from build123d import *

# Parameters (mm, degrees)
BOSS_EXTRUDE1_DEPTH = 50
BOSS_EXTRUDE2_DEPTH = 1.52
CUT_EXTRUDE2_DEPTH  = 1.52
CUT_EXTRUDE3_DEPTH  = 29
BOSS_EXTRUDE3_DEPTH = 1.55
SKETCH6_R           = 1
CUT_EXTRUDE4_DEPTH  = 77.55
CUT_EXTRUDE5_DEPTH  = 77.55
SKETCH8_R           = 1
CUT_EXTRUDE6_DEPTH  = 70
BOSS_EXTRUDE4_DEPTH = 1.5
BOSS_EXTRUDE5_DEPTH = 1.5
SKETCH12_R          = 10
CUT_EXTRUDE7_DEPTH  = 70


with BuildPart() as part:
    # Sketch1 → Boss-Extrude1 (new body)
    with BuildSketch(Plane(origin=(0, 0, 0), x_dir=(1, 0, 0), z_dir=(0, 1, 0))):
        Polygon((-22.935245878, -45.076760645), (20.864754122, -45.076760645), (20.864754122, 42.660744493), (4.698193973, 48.553690828), (4.698193973, 38.723239355), (-6.768685729, 38.723239355), (-6.768685729, 48.553690828), (-22.935245878, 42.660744493), align=None)
        Polygon((-21.435245878, -43.576760645), (19.364754122, -43.576760645), (19.364754122, 41.610970221), (6.198193973, 46.410372917), (6.198193973, 37.223239355), (-8.268685729, 37.223239355), (-8.268685729, 46.410372917), (-21.435245878, 41.610970221), align=None, mode=Mode.SUBTRACT)
    extrude(amount=BOSS_EXTRUDE1_DEPTH)

    # Sketch2 → Boss-Extrude2 (add)
    with BuildSketch(Plane(origin=(0, 50, 0), x_dir=(1, 0, 0), z_dir=(0, 1, 0))):
        Polygon((-22.935245878, 42.660744493), (-22.935245878, -45.076760645), (20.864754122, -45.076760645), (20.864754122, 42.660744493), (4.698193973, 48.553690828), (4.698193973, 38.723239355), (-6.768685729, 38.723239355), (-6.768685729, 48.553690828), align=None)
    extrude(amount=BOSS_EXTRUDE2_DEPTH)

    # Sketch3 → Cut-Extrude2 (cut)
    with BuildSketch(Plane.XY.offset(45.076760645)):
        with BuildLine():
            ThreePointArc((-11.035245878, 20), (-18.10631369, 17.071067812), (-21.035245878, 10))
            Line((-21.035245878, 10), (-21.035245878, 0))
            Line((-21.035245878, 0), (18.964754122, 0))
            Line((18.964754122, 0), (18.964754122, 10))
            ThreePointArc((18.964754122, 10), (16.035821934, 17.071067812), (8.964754122, 20))
            Line((8.964754122, 20), (-11.035245878, 20))
        make_face()
        with BuildLine():
            Line((-21.035245878, 0), (-21.035245878, 10))
            ThreePointArc((-21.035245878, 10), (-18.10631369, 17.071067812), (-11.035245878, 20))
            Line((-11.035245878, 20), (8.964754122, 20))
            ThreePointArc((8.964754122, 20), (16.035821934, 17.071067812), (18.964754122, 10))
            Line((18.964754122, 10), (18.964754122, 0))
            Line((18.964754122, 0), (19.264754122, 0))
            Line((19.264754122, 0), (19.264754122, 10))
            ThreePointArc((19.264754122, 10), (16.247953968, 17.283199846), (8.964754122, 20.3))
            Line((8.964754122, 20.3), (-11.035245878, 20.3))
            ThreePointArc((-11.035245878, 20.3), (-18.318445724, 17.283199846), (-21.335245878, 10))
            Line((-21.335245878, 10), (-21.335245878, 0))
            Line((-21.335245878, 0), (-21.035245878, 0))
        make_face()
    extrude(amount=-CUT_EXTRUDE2_DEPTH, mode=Mode.SUBTRACT)

    # Sketch4 → Cut-Extrude3 (cut)
    with BuildSketch(Plane(origin=(0, 51.52, 0), x_dir=(1, 0, 0), z_dir=(0, 1, 0))):
        Polygon((-6.768685729, 48.553690828), (-22.935245878, 42.660744493), (-22.935245878, -45.076760645), (20.864754122, -45.076760645), (20.864754122, 42.660744493), (4.698193973, 48.553690828), (4.698193973, 38.723239355), (-6.768685729, 38.723239355), align=None)
    extrude(amount=-CUT_EXTRUDE3_DEPTH, mode=Mode.SUBTRACT)

    # Sketch5 → Boss-Extrude3 (add)
    with BuildSketch(Plane(origin=(0, 22.52, 0), x_dir=(1, 0, 0), z_dir=(0, 1, 0))):
        Polygon((-6.768685729, 38.723239355), (-6.768685729, 48.553690828), (-22.935245878, 42.660744493), (-22.935245878, -45.076760645), (20.864754122, -45.076760645), (20.864754122, 42.660744493), (4.698193973, 48.553690828), (4.698193973, 38.723239355), align=None)
    extrude(amount=BOSS_EXTRUDE3_DEPTH)

    # Sketch6 → Cut-Extrude4 (cut)
    with BuildSketch(Plane(origin=(20.864754122, 0, 0), x_dir=(0, 0, -1), z_dir=(1, 0, 0))):
        with Locations((28.752953433, 10)):
            Circle(SKETCH6_R)
        with Locations((-29.280174862, 10)):
            Circle(SKETCH6_R)
    extrude(amount=-CUT_EXTRUDE4_DEPTH, mode=Mode.SUBTRACT)

    # Sketch7 → Cut-Extrude5 (cut)
    with BuildSketch(Plane(origin=(20.864754122, 0, 0), x_dir=(0, 0, -1), z_dir=(1, 0, 0))):
        Polygon((6.475840318, 5), (-8.89185647, 5), (-11.208008076, 2.683848394), (-11.208008076, 0), (8.791991924, 0), (8.791991924, 2.683848394), align=None)
    extrude(amount=-CUT_EXTRUDE5_DEPTH, mode=Mode.SUBTRACT)

    # Sketch8 → Cut-Extrude6 (cut)
    with BuildSketch(Plane(origin=(20.864754122, 0, 0), x_dir=(0, 0, -1), z_dir=(1, 0, 0))):
        with BuildLine():
            ThreePointArc((28.041256502, 10.702486639), (26.94988664, 10.925120784), (26.32955957, 10))
            Line((26.32955957, 10), (27.752953433, 10))
            ThreePointArc((27.752953433, 10), (27.827832649, 10.379672931), (28.041256502, 10.702486639))
        make_face()
        with BuildLine():
            Line((27.752953433, 10), (26.32955957, 10))
            ThreePointArc((26.32955957, 10), (26.94988664, 9.074879216), (28.041256502, 9.297513361))
            ThreePointArc((28.041256502, 9.297513361), (27.827832649, 9.620327069), (27.752953433, 10))
        make_face()
        with BuildLine():
            ThreePointArc((28.041256502, 10.702486639), (27.827832649, 10.379672931), (27.752953433, 10))
            Line((27.752953433, 10), (28.32955957, 10))
            ThreePointArc((28.32955957, 10), (28.254680355, 10.379672931), (28.041256502, 10.702486639))
        make_face()
        with BuildLine():
            Line((28.32955957, 10), (27.752953433, 10))
            ThreePointArc((27.752953433, 10), (27.827832649, 9.620327069), (28.041256502, 9.297513361))
            ThreePointArc((28.041256502, 9.297513361), (28.254680355, 9.620327069), (28.32955957, 10))
        make_face()
        with BuildLine():
            ThreePointArc((29.752953433, 10), (29.132626364, 10.925120784), (28.041256502, 10.702486639))
            ThreePointArc((28.041256502, 10.702486639), (28.254680355, 10.379672931), (28.32955957, 10))
            ThreePointArc((28.32955957, 10), (28.254680355, 9.620327069), (28.041256502, 9.297513361))
            ThreePointArc((28.041256502, 9.297513361), (29.132626364, 9.074879216), (29.752953433, 10))
        make_face()
        with Locations((-30.703568725, 10)):
            Circle(SKETCH8_R)
        with Locations((-29.280174862, 10)):
            Circle(SKETCH8_R)
    extrude(amount=-CUT_EXTRUDE6_DEPTH, mode=Mode.SUBTRACT)

    # Sketch10 → Boss-Extrude4 (add)
    with BuildSketch(Plane(origin=(20.864754122, 0, 0), x_dir=(0, 0, -1), z_dir=(1, 0, 0))):
        with BuildLine():
            ThreePointArc((-29.991871794, 9.297513361), (-28.280174862, 10), (-29.991871794, 10.702486639))
            ThreePointArc((-29.991871794, 10.702486639), (-29.778447941, 10.379672931), (-29.703568725, 10))
            ThreePointArc((-29.703568725, 10), (-29.778447941, 9.620327069), (-29.991871794, 9.297513361))
        make_face()
        with BuildLine():
            ThreePointArc((28.041256502, 10.702486639), (28.254680355, 10.379672931), (28.32955957, 10))
            ThreePointArc((28.32955957, 10), (28.254680355, 9.620327069), (28.041256502, 9.297513361))
            ThreePointArc((28.041256502, 9.297513361), (29.752953433, 10), (28.041256502, 10.702486639))
        make_face()
    extrude(amount=-BOSS_EXTRUDE4_DEPTH)

    # Sketch11 → Boss-Extrude5 (add)
    with BuildSketch(Plane.ZY.offset(22.935245878)):
        Polygon((-41.610970221, 22.52), (-41.610970221, 0), (-8.791991924, 0), (-8.791991924, 2.683848394), (-6.475840318, 5), (8.89185647, 5), (11.208008076, 2.683848394), (11.208008076, 0), (43.576760645, 0), (43.576760645, 22.52), align=None)
        with BuildLine():
            ThreePointArc((-28.041256502, 10.702486639), (-26.94988664, 10.925120784), (-26.32955957, 10))
            ThreePointArc((-26.32955957, 10), (-26.94988664, 9.074879216), (-28.041256502, 9.297513361))
            ThreePointArc((-28.041256502, 9.297513361), (-29.752953433, 10), (-28.041256502, 10.702486639))
        make_face(mode=Mode.SUBTRACT)
        with BuildLine():
            ThreePointArc((29.991871794, 10.702486639), (31.083241656, 10.925120784), (31.703568725, 10))
            ThreePointArc((31.703568725, 10), (31.083241656, 9.074879216), (29.991871794, 9.297513361))
            ThreePointArc((29.991871794, 9.297513361), (28.280174862, 10), (29.991871794, 10.702486639))
        make_face(mode=Mode.SUBTRACT)
        with BuildLine():
            ThreePointArc((29.991871794, 9.297513361), (29.703568725, 10), (29.991871794, 10.702486639))
            ThreePointArc((29.991871794, 10.702486639), (28.280174862, 10), (29.991871794, 9.297513361))
        make_face()
        with BuildLine():
            ThreePointArc((-28.041256502, 9.297513361), (-28.32955957, 10), (-28.041256502, 10.702486639))
            ThreePointArc((-28.041256502, 10.702486639), (-29.752953433, 10), (-28.041256502, 9.297513361))
        make_face()
    extrude(amount=-BOSS_EXTRUDE5_DEPTH)

    # Sketch12 → Cut-Extrude7 (cut)
    with BuildSketch(Plane(origin=(0, 24.07, 0), x_dir=(1, 0, 0), z_dir=(0, 1, 0))):
        with Locations(Location((-1.035245878, 12.363239355, 0), (0, 0, 270))):
            Circle(SKETCH12_R)
    extrude(amount=-CUT_EXTRUDE7_DEPTH, mode=Mode.SUBTRACT)


solid = part.part
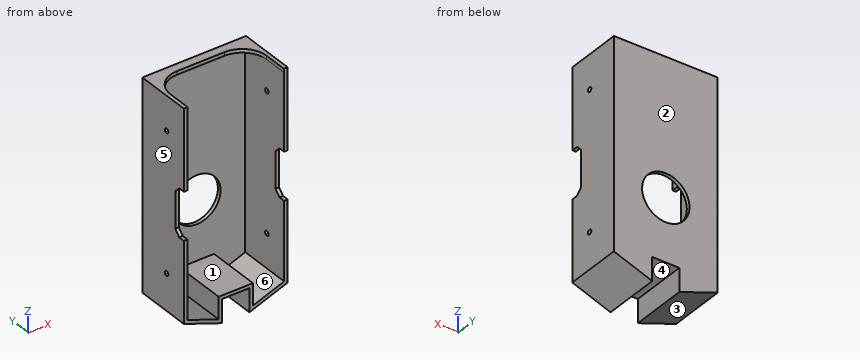
Part model, mm, in its own coordinate system. Face numbers are marked on the shaded views. A direction names the side the tool comes from. Round coordinates to 2 decimals unless told otherwise and drop trailing zeros. Order: outer loops, then holes, each group sorted by start corner. A loop starts at its lowest first (then second) coordinate and runs counter-clockwise, first axis right, second up. Notation, with made-up numbers: (-4.5, 74.25) -> (7.5, 74.25) arc R18 ccw to (7.5, 83.25) -> close; hole circle Ø7 at (-4.5, 16.25). An arc over 180 degrees is marked (long way). Put each result on its own line as item: value.
Q1. Pin check, flat tips, straight feed: pin 1 Ø1.2 at (x, z) = (20, 3.5) entering from -Y; pin 2 Ø11.5 at (x, y) = (0.5, 6.5) entering from +Z; pin 3 Ø10 at (y, z) = (17, -43.5) entering from +X; pin 4 Ø5 at (x, z) = (-17, -23) entering from -Y. Stop position of each tip, or through.
From the geometry:
pin 1: stops at y = 5
pin 2: stops at z = -37.22
pin 3: stops at x = 20.86
pin 4: stops at y = 22.52
Q2. Band-saw the part on D-D (x = 11). Give the cut face in (y, z).
From the geometry:
outline: (0, -46.26) -> (24.07, -46.26) -> (24.07, 45.08) -> (20.1, 45.08) -> (20.1, 43.58) -> (22.52, 43.58) -> (22.52, -44.66) -> (0, -44.66) -> close
Q3. Band-saw the part on B-B (z = -32). Give the cut face in (x, y), and give its area (3 significant figures).
From the geometry:
outline: (-22.94, 0) -> (-21.44, 0) -> (-21.44, 22.52) -> (19.36, 22.52) -> (19.36, 0) -> (20.86, 0) -> (20.86, 24.07) -> (-22.94, 24.07) -> close
area: 135 mm2
Q4. Wall check: line 1 (X direction, y = 15, z = 31); line 2 (Z direction, x = -22, y = 10); line 3 (Y direction, x = 10.5, z = 41). Give the ranges that are in metal, low to high. Write a range as [from, to].
From the geometry:
line 1: x = [-22.94, -21.44], [19.36, 20.86]
line 2: z = [-43, -28.33], [-26.33, 29.7], [31.7, 45.08]
line 3: y = [22.52, 24.07]
Q5. Tool access for the marked faces 4, 5 and 6: list every direction of +Z, -Z, +X, -X, +Y, -Y with a clear straight run to the whole face (end or side of a thin tool).
From the geometry:
face 4: -Z, +Y, -Y
face 5: +Z, -Z, -X, +Y, -Y
face 6: -Y
Q6. Band-saw the part on C-C (y = 14). Give the cut face in (x, z), and give its area (3 significant figures).
From the geometry:
outline: (-22.94, -42.66) -> (-6.77, -48.55) -> (-6.77, -38.72) -> (4.7, -38.72) -> (4.7, -48.55) -> (20.86, -42.66) -> (20.86, 45.08) -> (18.46, 45.08) -> (18.46, 43.58) -> (19.36, 43.58) -> (19.36, -41.61) -> (6.2, -46.41) -> (6.2, -37.22) -> (-8.27, -37.22) -> (-8.27, -46.41) -> (-21.44, -41.61) -> (-21.44, 43.58) -> (-20.53, 43.58) -> (-20.53, 45.08) -> (-22.94, 45.08) -> close
area: 359 mm2
Q7. Pull direction X, two halves, no side cores. Call the marked faces 1, 2 and 3: pulls with the +X half, pulls with the -X half, needs draft (parallel to the pull), parting line crosses it, or undercut.
From the geometry:
face 1: undercut
face 2: needs draft
face 3: pulls with the -X half
Q8. Band-saw the part on A-A (x = -4). Give the cut face in (y, z), and give its area (3 significant figures).
From the geometry:
outline: (0, -38.72) -> (24.07, -38.72) -> (24.07, -21.91) -> (22.52, -21.91) -> (22.52, -37.22) -> (0, -37.22) -> close; (20.3, 43.58) -> (22.52, 43.58) -> (22.52, -2.81) -> (24.07, -2.81) -> (24.07, 45.08) -> (20.3, 45.08) -> close
area: 137 mm2
